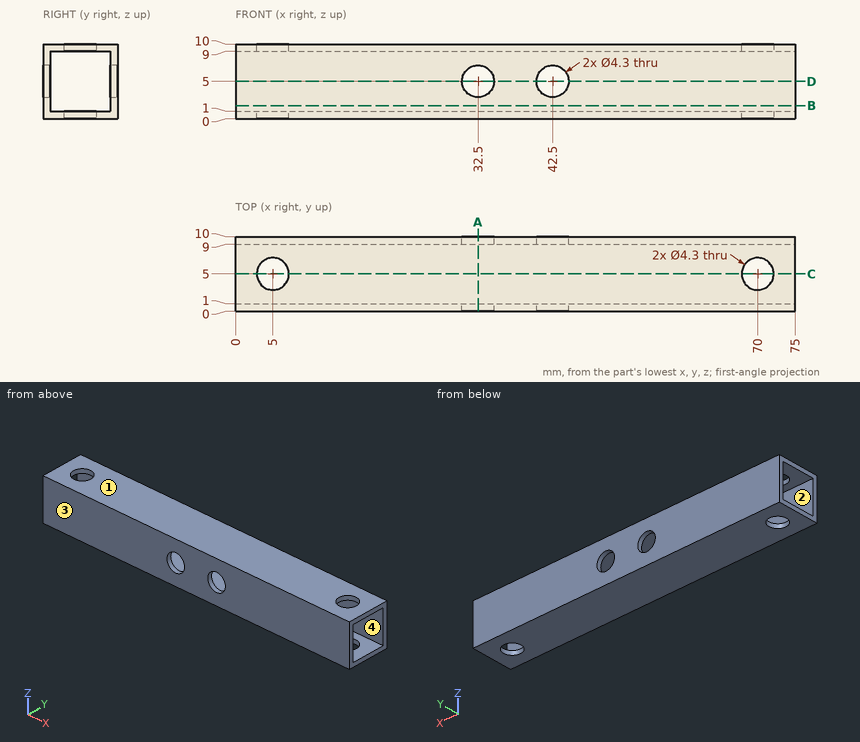
Print and shaded views of the part. All mm, measured from the part's lowest x, y and z. Coordinates: 2 decimals unless noted, no trailing zeros. Order: outer loops, then holes, each group sorted by start corner. A loop starts at its lowest first (then second) coordinate and runs counter-clockwise, first axis right, second up. Notation, with made-up numbers: (51.5, 36.25) -> (79.5, 36.25) arc R18 cw to (79.5, 56.25) -> close; hole circle Ø2 at (69.25, 12). An arc over 180 degrees is marked (long way). Answer as a JSON object with one key per item and string values. Group by question number.
1) Drill centre lines: L1, parallel to X at y = 0.5, z = 5; L2, parallel to Y at x = 29.5, z = 5. Where is each one in solid material? Low to high.
2) Cut at B-B, the plane z = 1.75. Write the cut outline in (x, y), then the cut area to 3 significant figures.
3) Pull direction Y, two halves, no side cores. Call the marked faces 1, 2, 3 and 4: +Y half, -Y half, draft (parallel to the pull), parting line (faces both ways), or undercut.
4) Cut at C-C, the plane y = 5. Write the cut outline in (x, z), then the cut area to 3 significant figures.
5) Flat gauge pin, fed straight in: pin 1 (3.5 mm diameter, centred on x = 42.5, z = 5, fed in from -Y). Where does the tip first touch, or does it go through?
6) Cut at A-A, the plane x = 32.5. Write the cut outline in (y, z), then the cut area to 3 significant figures.
7) Cut at D-D, the plane z = 5. Write the cut outline in (x, y), then the cut area to 3 significant figures.
Check values:
{
 "1": {"L1": "x = 0 to 30.35, 34.65 to 40.35, 44.65 to 75", "L2": "y = 0 to 1, 9 to 10"},
 "2": {"outline": "(0, 0) -> (75, 0) -> (75, 1) -> (0, 1) -> close; (0, 9) -> (75, 9) -> (75, 10) -> (0, 10) -> close", "area": "150 mm²"},
 "3": {"face 1": "draft", "face 2": "undercut", "face 3": "-Y half", "face 4": "undercut"},
 "4": {"outline": "(0, 0) -> (2.85, 0) -> (2.85, 1) -> (0, 1) -> close; (0, 9) -> (2.85, 9) -> (2.85, 10) -> (0, 10) -> close; (7.15, 0) -> (67.85, 0) -> (67.85, 1) -> (7.15, 1) -> close; (7.15, 9) -> (67.85, 9) -> (67.85, 10) -> (7.15, 10) -> close; (72.15, 0) -> (75, 0) -> (75, 1) -> (72.15, 1) -> close; (72.15, 9) -> (75, 9) -> (75, 10) -> (72.15, 10) -> close", "area": "133 mm²"},
 "5": {"pin 1": "passes through"},
 "6": {"outline": "(0, 0) -> (10, 0) -> (10, 2.85) -> (9, 2.85) -> (9, 1) -> (1, 1) -> (1, 2.85) -> (0, 2.85) -> close; (0, 7.15) -> (1, 7.15) -> (1, 9) -> (9, 9) -> (9, 7.15) -> (10, 7.15) -> (10, 10) -> (0, 10) -> close", "area": "27.4 mm²"},
 "7": {"outline": "(0, 0) -> (30.35, 0) -> (30.35, 1) -> (0, 1) -> close; (0, 9) -> (30.35, 9) -> (30.35, 10) -> (0, 10) -> close; (34.65, 0) -> (40.35, 0) -> (40.35, 1) -> (34.65, 1) -> close; (34.65, 9) -> (40.35, 9) -> (40.35, 10) -> (34.65, 10) -> close; (44.65, 0) -> (75, 0) -> (75, 1) -> (44.65, 1) -> close; (44.65, 9) -> (75, 9) -> (75, 10) -> (44.65, 10) -> close", "area": "133 mm²"}
}
